```python
from build123d import *

# Parameters (mm, degrees)
SKETCH_W        = 70.5
SKETCH_H        = 43.6
PAD_DEPTH       = 2.5
SKETCH001_W     = 60
SKETCH001_H     = 41
POCKET_DEPTH    = 1.8
SKETCH002_W     = 2.6
SKETCH002_H     = 18
POCKET001_DEPTH = 5


with BuildPart() as part:
    # Sketch → Pad (new body)
    with BuildSketch(Plane.XY):
        Rectangle(SKETCH_W, SKETCH_H)
    extrude(amount=PAD_DEPTH)

    # Sketch001 (on Face6 of Pad) → Pocket (cut)
    with BuildSketch(Plane.XY.offset(2.5)):
        Rectangle(SKETCH001_W, SKETCH001_H)
    extrude(amount=-POCKET_DEPTH, mode=Mode.SUBTRACT)

    # Sketch002 (on Face5 of Pocket) → Pocket001 (cut)
    with BuildSketch(Plane.XY.offset(2.5)):
        with Locations((33.95, 0)):
            Rectangle(SKETCH002_W, SKETCH002_H)
    extrude(amount=-POCKET001_DEPTH, mode=Mode.SUBTRACT)


solid = part.part
```
Source: CAD feature listing. Evaluate the final solid. Frame: model axes, mm. A direction names the side the tool comes from. Give positions to 0.01 mm unless a question says otherwise; leave off trailing zeros. Loops run counter-clockwise (first coordinate to the right, second up) from the corner with the lowest first, then second, coordinate; pieces in that order, holes last. Notation, with made-up numbers: (77, 67) -> (108, 67) arc R35 cw to (108, 101) -> close; hole circle Ø11 at (69.25, -25.75). An arc over 180 degrees is marked (long way). Put each result on its own line as item: value. Start each with the question number.
1) Material intervals for probe 1 along X at (y, z) = (19.5, 1.9); probe 2 along Y at (x, z) = (8.5, 0.75); probe 3 along X at (y, z) = (-3, 0.85), sorted ascending.
2) Contact query for flat-ended pins moving along their axis: P1, Ø4, axis at x = -14.5, y = 14.5, coming from the +Z side; P2, Ø0.8, axis at y = -2, z = 1, coming from the +X side. Output: stop coordinate, or through.
3) Draft query along X for faces 4 (the face through (0, -20.5, 2)), 5 (the face through (-35.25, 0, 1)), 6 (the face through (35.25, 15, 1)), 7 (the face through (0, 21.8, 1)). Return one class per face: released by +X, released by -X, zero draft, split by the parting line, or undercut.
4) Cut plane B-B (y = -8). Return loops of the section in (x, z), then the cut area to 4 significant figures.
5) Reachability of faces 1 (the face through (30, 0, 2)), 2 (the face through (0, -21.8, 1)), 3 (the face through (34, -9, 1)) from +Z, -Z, +X, -X, +Y, -Y: full face, straight path, thin tool, end or side. Return the list, or none.
6) Cut plane C-C (x = 28). Return loops of the section in (y, z).
7) Cut plane A-A (z = 1.4). Return loops of the section in (x, y).
Results are:
1. probe 1: x = -35.25 to -30, 30 to 35.25
1. probe 2: y = -21.8 to -20.5, 20.5 to 21.8
1. probe 3: x = -35.25 to -30, 30 to 32.65
2. P1: stops at z = 0.7
2. P2: stops at x = 32.65
3. face 4: undercut
3. face 5: released by -X
3. face 6: released by +X
3. face 7: zero draft
4. outline: (-35.25, 0) -> (32.65, 0) -> (32.65, 2.5) -> (30, 2.5) -> (30, 0.7) -> (-30, 0.7) -> (-30, 2.5) -> (-35.25, 2.5) -> close
4. area: 61.75 mm2
5. face 1: +Z
5. face 2: +Z, -Z, +X, -X, -Y
5. face 3: +Z, -Z, +X
6. outline: (-21.8, 0) -> (21.8, 0) -> (21.8, 2.5) -> (20.5, 2.5) -> (20.5, 0.7) -> (-20.5, 0.7) -> (-20.5, 2.5) -> (-21.8, 2.5) -> close
7. outline: (-35.25, -21.8) -> (35.25, -21.8) -> (35.25, -9) -> (32.65, -9) -> (32.65, 9) -> (35.25, 9) -> (35.25, 21.8) -> (-35.25, 21.8) -> close; hole (-30, -20.5) -> (30, -20.5) -> (30, 20.5) -> (-30, 20.5) -> close
